CAD build for the part. Positions are in the model's coordinates, mm. A direction names the side the tool comes from. Round coordinates to 2 decimals unless told otherwise and drop trailing zeros. Loops run counter-clockwise (first coordinate to the right, second up) from the corner with the lowest first, then second, coordinate; pieces in that order, holes last.
from build123d import *

# Parameters (mm, degrees)
SKETCH_R        = 7.5
PAD_DEPTH       = 70
SKETCH001_W     = 60
SKETCH001_H     = 48.25
POCKET_DEPTH    = 30
POCKET001_DEPTH = 50
POCKET002_DEPTH = 50
SKETCH004_W     = 10
SKETCH004_H     = 10
POCKET003_DEPTH = 5


with BuildPart() as part:
    # Sketch → Pad (new body)
    with BuildSketch(Plane.YZ):
        with BuildLine():
            ThreePointArc((-36.4599581718, 13.2911850247), (-57.9795050803, 3.5799598665), (-43.412972048, -15))
            Line((-43.412972048, -15), (41.5884017265, -15))
            ThreePointArc((41.5884017265, -15), (56.1336656173, 3.6654186747), (34.479804051, 13.2086275283))
            ThreePointArc((-36.4599581718, 13.2911850247), (-1.0004550601, 4.3323292657), (34.479804051, 13.2086275283))
        make_face()
        with Locations((-43.4129719528, 0)):
            Circle(SKETCH_R, mode=Mode.SUBTRACT)
    extrude(amount=PAD_DEPTH)

    # Sketch001 → Pocket (cut)
    with BuildSketch(Plane.XY.offset(15)):
        with Locations((35, 32.465)):
            Rectangle(SKETCH001_W, SKETCH001_H)
    extrude(amount=-POCKET_DEPTH, mode=Mode.SUBTRACT)

    # Sketch002 → Pocket001 (cut)
    with BuildSketch(Plane(origin=(3, -0.1, -20), x_dir=(1, 0, 0), z_dir=(0, 0, 1))):
        with BuildLine():
            ThreePointArc((17, -58.6013099487), (11.7906635923, -28.3224370767), (-3, -1.3932039145))
            Line((-3, -1.3932039145), (-3, -58.6013099487))
            Line((-3, -58.6013099487), (17, -58.6013099487))
        make_face()
        with BuildLine():
            ThreePointArc((67.0222612126, -1.66), (52.2953112485, -28.3670320419), (47, -58.4021497296))
            Line((66.999998461, -58.4099956332), (47, -58.4021497296))
            Line((67.0222612126, -1.66), (66.999998461, -58.4099956332))
        make_face()
    extrude(amount=POCKET001_DEPTH, mode=Mode.SUBTRACT)

    # Sketch003 → Pocket002 (cut)
    with BuildSketch(Plane.XY.offset(20)):
        with BuildLine():
            Line((10, -1.66), (60, -1.66))
            ThreePointArc((60, -1.66), (52.3618075612, -14.5061818768), (46.88, -28.41))
            Line((21.88, -28.41), (46.88, -28.41))
            ThreePointArc((21.88, -28.41), (16.9989570858, -14.5647042924), (10, -1.66))
        make_face()
    extrude(amount=-POCKET002_DEPTH, mode=Mode.SUBTRACT)

    # Sketch004 → Pocket003 (cut)
    with BuildSketch(Plane.YZ.offset(70)):
        with Locations((43.59, 0)):
            Rectangle(SKETCH004_W, SKETCH004_H)
    extrude(amount=-POCKET003_DEPTH, mode=Mode.SUBTRACT)


solid = part.part
Item 1: 3-axis set-ups, long thin cutter, end or side, ignore diameter. For faces 4 (the flat face through (35, -1.66, -5)), 5 (the flat face through (68, 44, 5)), 6 (the flat face through (5, 32, -3)), 7 (the cylindrical face through (34.785, -36.485, -2.873)), 8 (the flat face through (34.5, -1.5, -15)): which of +Z, -Z, +X, -X, +Y, -Y reach the whole face in a straight line?
Verdict:
face 4: +Z, -Z
face 5: +X
face 6: +Z, -Z, +Y
face 7: +X, -X
face 8: -Z, +X, -X, +Y, -Y
Item 2: Mould opens along X. For faces 1 (the cylindrical face through (55.448, -28.039, -3.527)), 2 (the cylindrical face through (2.465, 56.222, 3.294)), 3 (the flat face through (35, 8.34, -5)) say: released by +X, released by -X, zero draft, split by the parting line, or undercut.
Verdict:
face 1: released by +X
face 2: zero draft
face 3: undercut
Item 3: Cut at C-C (y = -26). List the corners of the cut face in (x, z).
Verdict:
outline: (13.91, -15) - (21.2, -15) - (21.2, 8.65) - (13.91, 8.65) - close; (47.65, -15) - (56.21, -15) - (56.21, 8.65) - (47.65, 8.65) - close
Item 4: Cut at B-B (z = 0). List the corners of the cut face in (x, y).
Verdict:
outline: (0, -1.49) arc R93 cw to (17.06, -35.91) - (53.01, -35.91) arc R93 cw to (70, -1.79) - (70, 38.59) - (65, 38.59) - (65, 8.34) - (5, 8.34) - (5, 56.59) - (0, 56.59) - close; (19.64, -50.91) arc R93 cw to (20, -58.41) - (50, -58.41) arc R93 cw to (50.38, -50.91) - close; (65, 48.59) - (70, 48.59) - (70, 56.59) - (65, 56.59) - close; hole (10, -1.66) arc R93 cw to (21.88, -28.41) - (46.88, -28.41) arc R93 cw to (60, -1.66) - close
Item 5: Cut at D-D (x = 54.5). List the corners of the cut face in (y, z), plus the area to 3 significant figures.
Verdict:
outline: (-30.82, -15) - (-10.41, -15) - (-10.41, 4.94) arc R75 cw to (-30.82, 10.55) - close; (-1.66, -15) - (8.34, -15) - (8.34, 4.91) arc R75 cw to (-1.66, 4.34) - close
area: 649 mm2
Item 6: Wall check: L1, parallel to Y at x = 26, z = 0; L2, parallel to X at y = 51.5, z = 6; L3, parallel to Y at x = 36, z = -5.5. Give the ranges that are in metal, low to high.
Verdict:
L1: y = -58.41 to -50.91, -35.91 to -28.41, -1.66 to 8.34
L2: x = 0 to 5, 65 to 70
L3: y = -57.37 to -48.51, -38.31 to -28.41, -1.66 to 8.34
Item 7: Cut at A-A (x = 41). List the corners of the cut face in (y, z).
Verdict:
outline: (-43.41, -15) - (-28.41, -15) - (-28.41, 9.55) arc R75 cw to (-36.46, 13.29) arc R15 ccw (long way) to start; (-1.66, -15) - (8.34, -15) - (8.34, 4.91) arc R75 cw to (-1.66, 4.34) - close; hole circle Ø15 at (-43.41, 0)
Item 8: Flat gauge pins, fed straight in: P1, Ø1.5, axis at x = 24.5, z = 8, coming from the +Y side; P2, Ø8, axis at x = 8, z = -7.5, coming from the -Y side; P3, Ø5, axis at x = 63, z = -5.5, coming from the +Y side; P4, Ø6, axis at x = 17.5, z = 1.5, coming from the -Y side. Where does each tip first touch, or does it go through?
Verdict:
P1: stops at y = -28.41
P2: stops at y = -21.38
P3: stops at y = 56.05
P4: stops at y = -58.41
